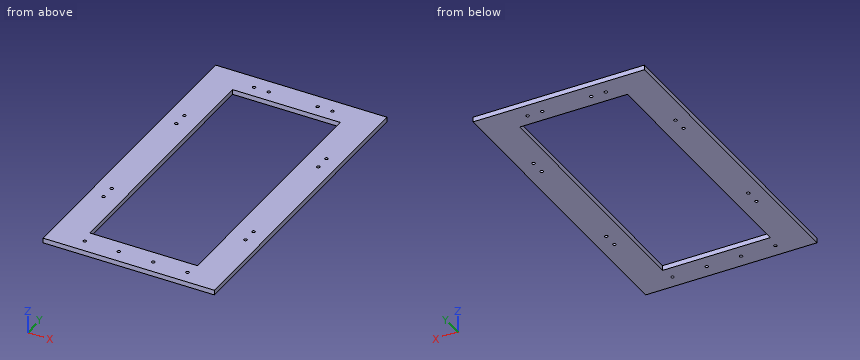
```python
from build123d import *

# Parameters (mm, degrees)
SKETCH1_W                      = 175
SKETCH1_H                      = 320
BOSS_EXTRUDE1_DEPTH            = 5
CUT_EXTRUDE1_REACH             = 7
SKETCH2_W                      = 110
SKETCH2_H                      = 265
CUT_EXTRUDE2_REACH             = 7
SKETCH4_R                      = 1.6
CUT_EXTRUDE3_REACH             = 7
SKETCH5_R                      = 1.6
CUT_EXTRUDE4_REACH             = 7
SKETCH6_R                      = 1.6
CUT_EXTRUDE4_DIRECTION_2_DEPTH = 1


with BuildPart() as part:
    # Sketch1 → Boss-Extrude1 (new body)
    with BuildSketch(Plane.XY):
        Rectangle(SKETCH1_W, SKETCH1_H)
    extrude(amount=BOSS_EXTRUDE1_DEPTH)

    # Sketch2 → Cut-Extrude1 (cut, up to next)
    with BuildSketch(Plane(origin=(0, 0, 0), x_dir=(-1, 0, 0), z_dir=(0, 0, -1)), mode=Mode.PRIVATE) as cut_extrude1_sk1:
        Rectangle(SKETCH2_W, SKETCH2_H)
    cut_extrude1_tool1 = extrude(cut_extrude1_sk1.sketch, amount=-CUT_EXTRUDE1_REACH, mode=Mode.PRIVATE) & part.part
    add(cut_extrude1_tool1.solids().sort_by_distance((0, 0, 0))[0], mode=Mode.SUBTRACT)

    # Sketch4 → Cut-Extrude2 (cut, up to next)
    with BuildSketch(Plane(origin=(0, 0, 0), x_dir=(-1, 0, 0), z_dir=(0, 0, -1)), mode=Mode.PRIVATE) as cut_extrude2_sk1:
        with Locations((-25, 145)):
            Circle(SKETCH4_R)
    cut_extrude2_tool1 = extrude(cut_extrude2_sk1.sketch, amount=-CUT_EXTRUDE2_REACH, mode=Mode.PRIVATE) & part.part
    add(cut_extrude2_tool1.solids().sort_by_distance((25, 145, 0))[0], mode=Mode.SUBTRACT)
    # Sketch4 → Cut-Extrude2 (cut, up to next)
    with BuildSketch(Plane(origin=(0, 0, 0), x_dir=(-1, 0, 0), z_dir=(0, 0, -1)), mode=Mode.PRIVATE) as cut_extrude2_sk2:
        with Locations((-40, 145)):
            Circle(SKETCH4_R)
    cut_extrude2_tool2 = extrude(cut_extrude2_sk2.sketch, amount=-CUT_EXTRUDE2_REACH, mode=Mode.PRIVATE) & part.part
    add(cut_extrude2_tool2.solids().sort_by_distance((40, 145, 0))[0], mode=Mode.SUBTRACT)
    # Sketch4 → Cut-Extrude2 (cut, up to next)
    with BuildSketch(Plane(origin=(0, 0, 0), x_dir=(-1, 0, 0), z_dir=(0, 0, -1)), mode=Mode.PRIVATE) as cut_extrude2_sk3:
        with Locations((25, 145)):
            Circle(SKETCH4_R)
    cut_extrude2_tool3 = extrude(cut_extrude2_sk3.sketch, amount=-CUT_EXTRUDE2_REACH, mode=Mode.PRIVATE) & part.part
    add(cut_extrude2_tool3.solids().sort_by_distance((-25, 145, 0))[0], mode=Mode.SUBTRACT)
    # Sketch4 → Cut-Extrude2 (cut, up to next)
    with BuildSketch(Plane(origin=(0, 0, 0), x_dir=(-1, 0, 0), z_dir=(0, 0, -1)), mode=Mode.PRIVATE) as cut_extrude2_sk4:
        with Locations((40, 145)):
            Circle(SKETCH4_R)
    cut_extrude2_tool4 = extrude(cut_extrude2_sk4.sketch, amount=-CUT_EXTRUDE2_REACH, mode=Mode.PRIVATE) & part.part
    add(cut_extrude2_tool4.solids().sort_by_distance((-40, 145, 0))[0], mode=Mode.SUBTRACT)

    # Sketch5 → Cut-Extrude3 (cut, up to next)
    with BuildSketch(Plane(origin=(0, 0, 0), x_dir=(-1, 0, 0), z_dir=(0, 0, -1)), mode=Mode.PRIVATE) as cut_extrude3_sk1:
        with Locations((-72.5, 75)):
            Circle(SKETCH5_R)
    cut_extrude3_tool1 = extrude(cut_extrude3_sk1.sketch, amount=-CUT_EXTRUDE3_REACH, mode=Mode.PRIVATE) & part.part
    add(cut_extrude3_tool1.solids().sort_by_distance((72.5, 75, 0))[0], mode=Mode.SUBTRACT)
    # Sketch5 → Cut-Extrude3 (cut, up to next)
    with BuildSketch(Plane(origin=(0, 0, 0), x_dir=(-1, 0, 0), z_dir=(0, 0, -1)), mode=Mode.PRIVATE) as cut_extrude3_sk2:
        with Locations((-72.5, 60)):
            Circle(SKETCH5_R)
    cut_extrude3_tool2 = extrude(cut_extrude3_sk2.sketch, amount=-CUT_EXTRUDE3_REACH, mode=Mode.PRIVATE) & part.part
    add(cut_extrude3_tool2.solids().sort_by_distance((72.5, 60, 0))[0], mode=Mode.SUBTRACT)
    # Sketch5 → Cut-Extrude3 (cut, up to next)
    with BuildSketch(Plane(origin=(0, 0, 0), x_dir=(-1, 0, 0), z_dir=(0, 0, -1)), mode=Mode.PRIVATE) as cut_extrude3_sk3:
        with Locations((-72.5, -75)):
            Circle(SKETCH5_R)
    cut_extrude3_tool3 = extrude(cut_extrude3_sk3.sketch, amount=-CUT_EXTRUDE3_REACH, mode=Mode.PRIVATE) & part.part
    add(cut_extrude3_tool3.solids().sort_by_distance((72.5, -75, 0))[0], mode=Mode.SUBTRACT)
    # Sketch5 → Cut-Extrude3 (cut, up to next)
    with BuildSketch(Plane(origin=(0, 0, 0), x_dir=(-1, 0, 0), z_dir=(0, 0, -1)), mode=Mode.PRIVATE) as cut_extrude3_sk4:
        with Locations((-72.5, -60)):
            Circle(SKETCH5_R)
    cut_extrude3_tool4 = extrude(cut_extrude3_sk4.sketch, amount=-CUT_EXTRUDE3_REACH, mode=Mode.PRIVATE) & part.part
    add(cut_extrude3_tool4.solids().sort_by_distance((72.5, -60, 0))[0], mode=Mode.SUBTRACT)
    # Sketch5 → Cut-Extrude3 (cut, up to next)
    with BuildSketch(Plane(origin=(0, 0, 0), x_dir=(-1, 0, 0), z_dir=(0, 0, -1)), mode=Mode.PRIVATE) as cut_extrude3_sk5:
        with Locations((72.5, -75)):
            Circle(SKETCH5_R)
    cut_extrude3_tool5 = extrude(cut_extrude3_sk5.sketch, amount=-CUT_EXTRUDE3_REACH, mode=Mode.PRIVATE) & part.part
    add(cut_extrude3_tool5.solids().sort_by_distance((-72.5, -75, 0))[0], mode=Mode.SUBTRACT)
    # Sketch5 → Cut-Extrude3 (cut, up to next)
    with BuildSketch(Plane(origin=(0, 0, 0), x_dir=(-1, 0, 0), z_dir=(0, 0, -1)), mode=Mode.PRIVATE) as cut_extrude3_sk6:
        with Locations((72.5, -60)):
            Circle(SKETCH5_R)
    cut_extrude3_tool6 = extrude(cut_extrude3_sk6.sketch, amount=-CUT_EXTRUDE3_REACH, mode=Mode.PRIVATE) & part.part
    add(cut_extrude3_tool6.solids().sort_by_distance((-72.5, -60, 0))[0], mode=Mode.SUBTRACT)
    # Sketch5 → Cut-Extrude3 (cut, up to next)
    with BuildSketch(Plane(origin=(0, 0, 0), x_dir=(-1, 0, 0), z_dir=(0, 0, -1)), mode=Mode.PRIVATE) as cut_extrude3_sk7:
        with Locations((72.5, 60)):
            Circle(SKETCH5_R)
    cut_extrude3_tool7 = extrude(cut_extrude3_sk7.sketch, amount=-CUT_EXTRUDE3_REACH, mode=Mode.PRIVATE) & part.part
    add(cut_extrude3_tool7.solids().sort_by_distance((-72.5, 60, 0))[0], mode=Mode.SUBTRACT)
    # Sketch5 → Cut-Extrude3 (cut, up to next)
    with BuildSketch(Plane(origin=(0, 0, 0), x_dir=(-1, 0, 0), z_dir=(0, 0, -1)), mode=Mode.PRIVATE) as cut_extrude3_sk8:
        with Locations((72.5, 75)):
            Circle(SKETCH5_R)
    cut_extrude3_tool8 = extrude(cut_extrude3_sk8.sketch, amount=-CUT_EXTRUDE3_REACH, mode=Mode.PRIVATE) & part.part
    add(cut_extrude3_tool8.solids().sort_by_distance((-72.5, 75, 0))[0], mode=Mode.SUBTRACT)

    # Sketch6 → Cut-Extrude4 (cut, up to next)
    with BuildSketch(Plane(origin=(0, 0, 0), x_dir=(-1, 0, 0), z_dir=(0, 0, -1)), mode=Mode.PRIVATE) as cut_extrude4_sk1:
        with Locations((52.5, -146.25)):
            Circle(SKETCH6_R)
    cut_extrude4_tool1 = extrude(cut_extrude4_sk1.sketch, amount=-CUT_EXTRUDE4_REACH, mode=Mode.PRIVATE) & part.part
    add(cut_extrude4_tool1.solids().sort_by_distance((-52.5, -146.25, 0))[0], mode=Mode.SUBTRACT)
    # Sketch6 → Cut-Extrude4 (cut, up to next)
    with BuildSketch(Plane(origin=(0, 0, 0), x_dir=(-1, 0, 0), z_dir=(0, 0, -1)), mode=Mode.PRIVATE) as cut_extrude4_sk2:
        with Locations((17.5, -146.25)):
            Circle(SKETCH6_R)
    cut_extrude4_tool2 = extrude(cut_extrude4_sk2.sketch, amount=-CUT_EXTRUDE4_REACH, mode=Mode.PRIVATE) & part.part
    add(cut_extrude4_tool2.solids().sort_by_distance((-17.5, -146.25, 0))[0], mode=Mode.SUBTRACT)
    # Sketch6 → Cut-Extrude4 (cut, up to next)
    with BuildSketch(Plane(origin=(0, 0, 0), x_dir=(-1, 0, 0), z_dir=(0, 0, -1)), mode=Mode.PRIVATE) as cut_extrude4_sk3:
        with Locations((-17.5, -146.25)):
            Circle(SKETCH6_R)
    cut_extrude4_tool3 = extrude(cut_extrude4_sk3.sketch, amount=-CUT_EXTRUDE4_REACH, mode=Mode.PRIVATE) & part.part
    add(cut_extrude4_tool3.solids().sort_by_distance((17.5, -146.25, 0))[0], mode=Mode.SUBTRACT)
    # Sketch6 → Cut-Extrude4 (cut, up to next)
    with BuildSketch(Plane(origin=(0, 0, 0), x_dir=(-1, 0, 0), z_dir=(0, 0, -1)), mode=Mode.PRIVATE) as cut_extrude4_sk4:
        with Locations((-52.5, -146.25)):
            Circle(SKETCH6_R)
    cut_extrude4_tool4 = extrude(cut_extrude4_sk4.sketch, amount=-CUT_EXTRUDE4_REACH, mode=Mode.PRIVATE) & part.part
    add(cut_extrude4_tool4.solids().sort_by_distance((52.5, -146.25, 0))[0], mode=Mode.SUBTRACT)

    # Sketch6 → Cut-Extrude4 direction 2 (cut)
    with BuildSketch(Plane(origin=(0, 0, 0), x_dir=(-1, 0, 0), z_dir=(0, 0, -1))):
        with Locations((52.5, -146.25)):
            Circle(SKETCH6_R)
        with Locations((17.5, -146.25)):
            Circle(SKETCH6_R)
        with Locations((-17.5, -146.25)):
            Circle(SKETCH6_R)
        with Locations((-52.5, -146.25)):
            Circle(SKETCH6_R)
    extrude(amount=CUT_EXTRUDE4_DIRECTION_2_DEPTH, mode=Mode.SUBTRACT)


solid = part.part
```
The listing builds one solid part. Answer for the finished solid, in the listing's coordinates (mm). Give positions to 0.01 mm unless a question says otherwise; leave off trailing zeros. Order: outer loops, then holes, each group sorted by start corner. A loop starts at its lowest first (then second) coordinate and runs counter-clockwise, first axis right, second up. Notation, with made-up numbers: (55, 60) - (108, 60) arc R15 cw to (108, 87) - close; hole circle Ø11 at (35, -26.5). An arc over 180 degrees is marked (long way). Answer in a Markdown table with one row per item. Add a question column.
Q1. The part is cut by section C-C (x = 5). Determine the outline of the cut face in (y, z).
Q2. Given P1, Ø3, axis at x = -52.5, y = -146.25, coming from the +Z side, flat-ended and moving along its own axis, determine where the tip first touches the part or whether it passes through.
Q3. The part is cut by section B-B (z = 3.2). Give the number of separate pieces and of enclosed holes in the cut face, then the cut area to 3 significant figures.
Q4. Find the intervals of material crossed by line 1 along Y through (x, z) = (52.5, 1.9); line 2 along Y through (x, z) = (25, 1.35); line 3 along X through (y, z) = (-146.25, 2.6), in increasing order. Write a range as [from, to].
Q5. The part is cut by section A-A (y = -126). Determine the outline of the cut face in (x, z), then the cut area to 3 significant figures.
Determined:
| question | item | result |
|---|---|---|
| 1 | outline | (-160, 0) - (-132.5, 0) - (-132.5, 5) - (-160, 5) - close; (132.5, 0) - (160, 0) - (160, 5) - (132.5, 5) - close |
| 2 | P1 | passes through |
| 3 | separate pieces | 1 |
| 3 | enclosed holes | 17 |
| 3 | area | 26,700 mm² |
| 4 | line 1 | y = [-160, -147.85], [-144.65, -132.5], [132.5, 160] |
| 4 | line 2 | y = [-160, -132.5], [132.5, 143.4], [146.6, 160] |
| 4 | line 3 | x = [-87.5, -54.1], [-50.9, -19.1], [-15.9, 15.9], [19.1, 50.9], [54.1, 87.5] |
| 5 | outline | (-87.5, 0) - (-55, 0) - (-55, 5) - (-87.5, 5) - close; (55, 0) - (87.5, 0) - (87.5, 5) - (55, 5) - close |
| 5 | area | 325 mm² |
